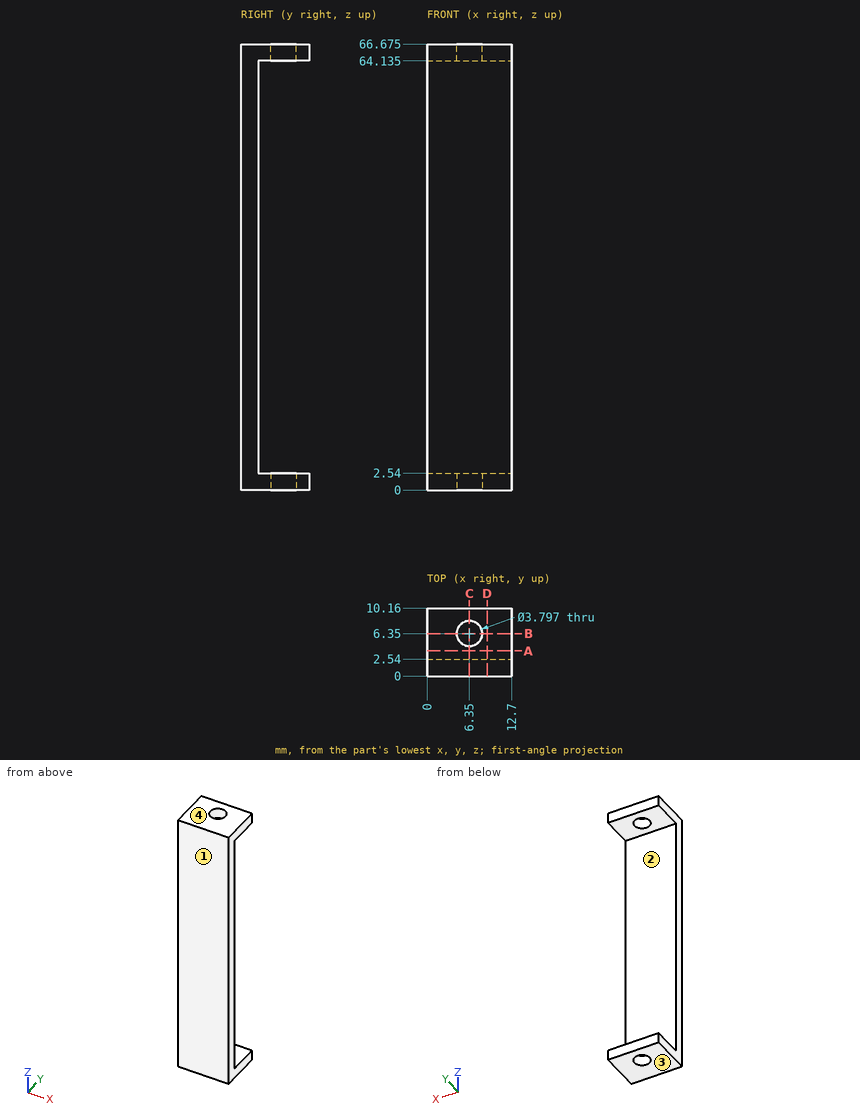
Verification items for this drawing (mm, ordinates from the low corner). Give positions to 0.01 mm unless a question says otherwise; leave off trailing zeros. Loops run counter-clockwise (first coordinate to the right, second up) from the corner with the lowest first, then second, coordinate; pieces in that order, holes last. Notation, with made-up numbers: M -24.75,69 L -12.75,69 A27 ccw -12.75,102 Z; hole C 84,66.5 d4. An arc over 180 degrees is marked long. Return JSON: item names as keys, results as strings. Group by question number.
1. Cross-section at A-A on y = 3.75. Record the boundary of the cut face in (x, z) (1 decimal).
2. Thickness scan on L1, parallel to Z at x = 5.75, y = 3.75 (1 decimal); L2, parallel to Y at x = 6.35, z = 1.85; L3, parallel to Y at x = 3, z = 30. Record the ranges inside material, lowest first.
3. Cross-section at D-D on x = 9. Record the boundary of the cut face in (y, z) (1 decimal), plus the area to 3 significant figures.
4. Cross-section at C-C on x = 6.35. Record the boundary of the cut face in (y, z) (1 decimal), plus the area to 3 significant figures.
5. Go/stop test with a flat-tipped pin: pin 1 (5 mm diameter, centred on x = 1.5, z = 22.5, fed in from +Y). Record where the tip stops, or that it passes through.
6. Mould release check, pull along Z, two halves, no side actions. Record for the marked faces 1, 2, 3 and 4: released by +Z, released by -Z, zero draft, split by the parting line, or undercut.
7. Cross-section at B-B on y = 6.35. Record the boundary of the cut face in (x, z) (1 decimal).
Return value:
{
 "1": {"outline": "M 0,0 L 12.7,0 L 12.7,2.5 L 0,2.5 Z; M 0,64.1 L 12.7,64.1 L 12.7,66.7 L 0,66.7 Z"},
 "2": {"L1": "0 to 2.5, 64.1 to 66.7", "L2": "0 to 4.45, 8.25 to 10.16", "L3": "0 to 2.54"},
 "3": {"outline": "M 0,0 L 10.2,0 L 10.2,2.5 L 2.5,2.5 L 2.5,64.1 L 10.2,64.1 L 10.2,66.7 L 0,66.7 Z", "area": "208 mm^2"},
 "4": {"outline": "M 0,0 L 4.5,0 L 4.5,2.5 L 2.5,2.5 L 2.5,64.1 L 4.5,64.1 L 4.5,66.7 L 0,66.7 Z; M 8.2,0 L 10.2,0 L 10.2,2.5 L 8.2,2.5 Z; M 8.2,64.1 L 10.2,64.1 L 10.2,66.7 L 8.2,66.7 Z", "area": "189 mm^2"},
 "5": {"pin 1": "y = 2.54"},
 "6": {"face 1": "zero draft", "face 2": "undercut", "face 3": "released by -Z", "face 4": "released by +Z"},
 "7": {"outline": "M 0,0 L 4.5,0 L 4.5,2.5 L 0,2.5 Z; M 0,64.1 L 4.5,64.1 L 4.5,66.7 L 0,66.7 Z; M 8.2,0 L 12.7,0 L 12.7,2.5 L 8.2,2.5 Z; M 8.2,64.1 L 12.7,64.1 L 12.7,66.7 L 8.2,66.7 Z"}
}
